Source: CAD feature listing. Evaluate the final solid. Frame: model axes, mm. A direction names the side the tool comes from. Give positions to 0.01 mm unless a question says otherwise; leave off trailing zeros. Loops run counter-clockwise (first coordinate to the right, second up) from the corner with the lowest first, then second, coordinate; pieces in that order, holes last. Notation, with made-up numbers: (57.25, 66.5) -> (65.25, 66.5) arc R21 ccw to (65.25, 70.5) -> close; hole circle Ø3 at (23, 21). An arc over 180 degrees is marked (long way). Return JSON: item names as keys, results as strings. Group by question number.
(1) Pin query (flat end, axial travel): pin 1 (6 mm diameter, centred on x = 14, y = -29.5, fed in from -Z); pin 2 (1 mm diameter, centred on y = -35.5, z = 4, fed in from -X); pin 3 (5 mm diameter, centred on x = 4, z = 8.5, fed in from -Y); pin 4 (10 mm diameter, centred on x = -2.5, y = -76, fed in from -Z). Return the tip coordinate at first contact, or that it passes through.
(2) Cut plane B-B on x = 0. Return loops of the section in (y, z), then the cut area to 3 significant figures.
(3) Cut plane C-C on z = 7.25. Return loops of the section in (x, y), then the cut area to 3 significant figures.
(4) Ray query, line 1 (Y direction, x = 2.25, z = 7.5); line 2 (X direction, y = -80, z = 6.25); line 3 (Y direction, x = -1.5, z = 6). Return the intervals inside material, ascending. Write a range as from..to.
(5) Draft query along Y for faces 1 (the face through (5.5, -79.9, 4.9)), 2 (the face through (3.8, -110, 3)), 3 (the face through (12, -108, 9)), 4 (the face through (14.997, -128.859, 9.493)). Return one class per face: released by +Y, released by -Y, zero draft, split by the parting line, or undercut.
(6) Cut plane A-A on y = -80. Return loops of the section in (x, z).
(7) Cut plane D-D on y = -16. Return loops of the section in (x, z), then the cut area to 3 significant figures.
(8) Access query for faces 5 (the face through (7, -43, 9)), 6 (the face through (5.23, -20.18, 7.5)), 7 (the face through (-3.8, -64, 5)). Directions: +Z, -Z, +X, -X, +Y, -Y. A direction counts if a zero-diameter tool reaches every point of the face in a straight line with its end or side. Return the directions, or none.
```python
from build123d import *

# Parameters (mm, degrees)
SKETCH1_R            = 2.5
BOSS_EXTRUDE1_DEPTH  = 10
SKETCH4_W            = 20
SKETCH4_H            = 45
BOSS_EXTRUDE2_DEPTH  = 1
FILLET3_R            = 0.8
FILLET2_R            = 4
FILLET1_R            = 5
FILLET3_OF_MIRROR1_R = 0.8
FILLET2_OF_MIRROR1_R = 4
FILLET1_OF_MIRROR1_R = 5


with BuildPart() as part:
    # Sketch1 → Boss-Extrude1 (new body)
    with BuildSketch(Plane.XY):
        with BuildLine():
            Line((-3.8, 6), (-3.8, -44.02382093))
            ThreePointArc((-3.8, -44.02382093), (-5.5, -48), (-3.8, -51.97617907))
            Line((-3.8, -51.97617907), (-3.8, -64))
            Line((-3.8, -64), (3.8, -64))
            Line((3.8, -64), (3.8, -51.97617907))
            ThreePointArc((3.8, -51.97617907), (5.5, -48), (3.8, -44.02382093))
            Line((3.8, -44.02382093), (3.8, 6))
            ThreePointArc((3.8, 6), (0, 13.252645761), (-3.8, 6))
        make_face()
        with Locations((0, -48)):
            Circle(SKETCH1_R, mode=Mode.SUBTRACT)
    boss_extrude1 = extrude(amount=BOSS_EXTRUDE1_DEPTH)

    # Sketch4 → Boss-Extrude2 (add)
    with BuildSketch(Plane.XY.offset(10)):
        with Locations((6.2, -20.5)):
            Rectangle(SKETCH4_W, SKETCH4_H)
    boss_extrude2 = extrude(amount=-BOSS_EXTRUDE2_DEPTH)

    # Fillet3
    fillet3_edges = [part.edges().sort_by_distance(p)[0] for p in [
        (0, 13.252645761, 0),
        (0, 13.252645761, 10),
    ]]
    fillet(fillet3_edges, radius=FILLET3_R)

    # Fillet2
    fillet2_edges = [part.edges().sort_by_distance(p)[0] for p in [
        (16.2, -43, 9.5),
        (16.2, 2, 9.5),
    ]]
    fillet(fillet2_edges, radius=FILLET2_R)

    # Fillet1
    fillet1_edges = [part.edges().sort_by_distance(p)[0] for p in [
        (3.8, -20.5, 9),
    ]]
    fillet(fillet1_edges, radius=FILLET1_R)

    # Mirror1: Boss-Extrude1, Boss-Extrude2 across plane
    add(boss_extrude1.mirror(Plane(origin=(0, -64, 0), x_dir=(0, 0, 1), z_dir=(0, -1, 0))))
    add(boss_extrude2.mirror(Plane(origin=(0, -64, 0), x_dir=(0, 0, 1), z_dir=(0, -1, 0))))

    # Fillet3 of Mirror1
    fillet3_of_mirror1_edges = [part.edges().sort_by_distance(p)[0] for p in [
        (0, -141.252645761, 0),
        (0, -141.252645761, 10),
    ]]
    fillet(fillet3_of_mirror1_edges, radius=FILLET3_OF_MIRROR1_R)

    # Fillet2 of Mirror1
    fillet2_of_mirror1_edges = [part.edges().sort_by_distance(p)[0] for p in [
        (16.2, -85, 9.5),
        (16.2, -130, 9.5),
    ]]
    fillet(fillet2_of_mirror1_edges, radius=FILLET2_OF_MIRROR1_R)

    # Fillet1 of Mirror1
    fillet1_of_mirror1_edges = [part.edges().sort_by_distance(p)[0] for p in [
        (3.8, -107.5, 9),
    ]]
    fillet(fillet1_of_mirror1_edges, radius=FILLET1_OF_MIRROR1_R)


solid = part.part
```
Answers:
{
 "1": {"pin 1": "z = 9", "pin 2": "x = -3.8", "pin 3": "y = -141", "pin 4": "z = 0"},
 "2": {"outline": "(-141.25, 0.8) arc R0.8 ccw to (-140.45, 0) -> (-82.5, 0) -> (-82.5, 10) -> (-140.45, 10) arc R0.8 ccw to (-141.25, 9.2) -> close; (-77.5, 0) -> (-50.5, 0) -> (-50.5, 10) -> (-77.5, 10) -> close; (-45.5, 0) -> (12.45, 0) arc R0.8 ccw to (13.25, 0.8) -> (13.25, 9.2) arc R0.8 ccw to (12.45, 10) -> (-45.5, 10) -> close", "area": "1,440 mm²"},
 "3": {"outline": "(-3.8, -134) arc R4.62 ccw (long way) to (3.8, -134) -> (3.8, -130) -> (5, -130) -> (5, -85) -> (3.8, -85) -> (3.8, -83.98) arc R5.5 ccw to (3.8, -76.02) -> (3.8, -51.98) arc R5.5 ccw to (3.8, -44.02) -> (3.8, -43) -> (5, -43) -> (5, 2) -> (3.8, 2) -> (3.8, 6) arc R4.62 ccw (long way) to (-3.8, 6) -> (-3.8, -44.02) arc R5.5 ccw to (-3.8, -51.98) -> (-3.8, -76.02) arc R5.5 ccw to (-3.8, -83.98) -> close; hole circle Ø5 at (0, -80); hole circle Ø5 at (0, -48)", "area": "1,280 mm²"},
 "4": {"line 1": "-140.67..-81.09, -78.91..-49.09, -46.91..12.67", "line 2": "-5.5..-2.5, 2.5..5.5", "line 3": "-141..-82, -78..-50, -46..13"},
 "5": {"face 1": "undercut", "face 2": "undercut", "face 3": "zero draft", "face 4": "released by -Y"},
 "6": {"outline": "(-5.5, 0) -> (-2.5, 0) -> (-2.5, 10) -> (-5.5, 10) -> close; (2.5, 0) -> (5.5, 0) -> (5.5, 10) -> (2.5, 10) -> close"},
 "7": {"outline": "(-3.8, 0) -> (3.8, 0) -> (3.8, 4) arc R5 cw to (8.8, 9) -> (16.2, 9) -> (16.2, 10) -> (-3.8, 10) -> close", "area": "93.8 mm²"},
 "8": {"face 5": "+Z, -Z, +X", "face 6": "-Z, +X", "face 7": "+Z, -Z, -X"}
}
